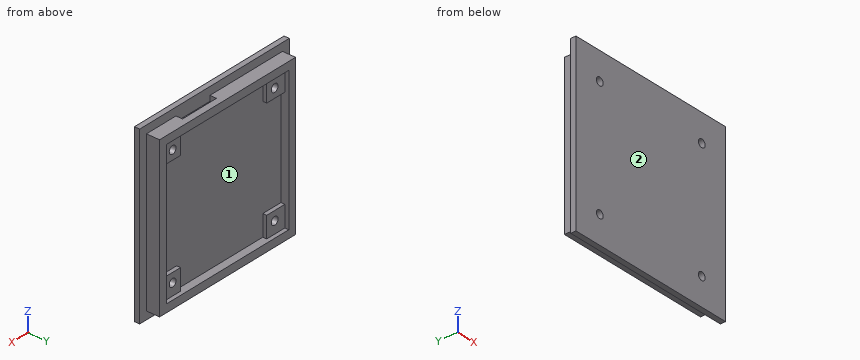
from build123d import *

# Parameters (mm, degrees)
SKETCH1_W           = 60
SKETCH1_H           = 60
BOSS_EXTRUDE1_DEPTH = 5
SKETCH2_W           = 54
SKETCH2_H           = 54
CUT_EXTRUDE1_DEPTH  = 3
SKETCH5_W           = 15
SKETCH5_H           = 2.5
CUT_EXTRUDE3_DEPTH  = 2
SKETCH6_W           = 12
SKETCH6_H           = 2
CUT_EXTRUDE4_DEPTH  = 2
SKETCH7_W           = 66
SKETCH7_H           = 66
BOSS_EXTRUDE3_DEPTH = 2
SKETCH4_W           = 8
SKETCH4_H           = 8
BOSS_EXTRUDE2_DEPTH = 1.5
SKETCH3_R           = 1.5
CUT_EXTRUDE2_DEPTH  = 5.5


with BuildPart() as part:
    # Sketch1 → Boss-Extrude1 (new body)
    with BuildSketch(Plane(origin=(0, 0, 0), x_dir=(1, 0, 0), z_dir=(0, 1, 0))):
        Rectangle(SKETCH1_W, SKETCH1_H)
    extrude(amount=BOSS_EXTRUDE1_DEPTH)

    # Sketch2 → Cut-Extrude1 (cut)
    with BuildSketch(Plane(origin=(0, 5, 0), x_dir=(1, 0, 0), z_dir=(0, 1, 0))):
        Rectangle(SKETCH2_W, SKETCH2_H)
    extrude(amount=-CUT_EXTRUDE1_DEPTH, mode=Mode.SUBTRACT)

    # Sketch5 → Cut-Extrude3 (cut)
    with BuildSketch(Plane(origin=(0, 0, 30), x_dir=(-1, 0, 0), z_dir=(0, 0, -1))):
        with Locations((-9.5, 1.25)):
            Rectangle(SKETCH5_W, SKETCH5_H)
    extrude(amount=CUT_EXTRUDE3_DEPTH, mode=Mode.SUBTRACT)

    # Sketch6 → Cut-Extrude4 (cut)
    with BuildSketch(Plane(origin=(0, 0, -30), x_dir=(-1, 0, 0), z_dir=(0, 0, -1))):
        with Locations((-17.5, 1)):
            Rectangle(SKETCH6_W, SKETCH6_H)
    extrude(amount=-CUT_EXTRUDE4_DEPTH, mode=Mode.SUBTRACT)

    # Sketch7 → Boss-Extrude3 (add)
    with BuildSketch(Plane.XZ):
        Rectangle(SKETCH7_W, SKETCH7_H)
    extrude(amount=BOSS_EXTRUDE3_DEPTH)

    # Sketch4 → Boss-Extrude2 (add)
    with BuildSketch(Plane(origin=(0, 2, 0), x_dir=(1, 0, 0), z_dir=(0, 1, 0))):
        with Locations((23, 23)):
            Rectangle(SKETCH4_W, SKETCH4_H)
        with Locations((-23, 23)):
            Rectangle(SKETCH4_W, SKETCH4_H)
        with Locations((23, -23)):
            Rectangle(SKETCH4_W, SKETCH4_H)
        with Locations((-23, -23)):
            Rectangle(SKETCH4_W, SKETCH4_H)
    extrude(amount=BOSS_EXTRUDE2_DEPTH)

    # Sketch3 → Cut-Extrude2 (cut)
    with BuildSketch(Plane(origin=(0, 3.5, 0), x_dir=(1, 0, 0), z_dir=(0, 1, 0))):
        with Locations(Location((-22.5, 22.5, 0), (0, 0, 270))):
            Circle(SKETCH3_R)
        with Locations(Location((22.5, 22.5, 0), (0, 0, 270))):
            Circle(SKETCH3_R)
        with Locations(Location((22.5, -22.5, 0), (0, 0, 270))):
            Circle(SKETCH3_R)
        with Locations(Location((-22.5, -22.5, 0), (0, 0, 270))):
            Circle(SKETCH3_R)
    extrude(amount=-CUT_EXTRUDE2_DEPTH, mode=Mode.SUBTRACT)


solid = part.part
Geometry check sheet. Reference: the model listing, model coordinates, mm. Face numbers are marked on the shaded views. Round coordinates to 2 decimals unless told otherwise and drop trailing zeros. Loops run counter-clockwise (first coordinate to the right, second up) from the corner with the lowest first, then second, coordinate; pieces in that order, holes last. Notation, with made-up numbers: (3.5, 89) - (11.5, 89) arc R33 cw to (11.5, 123) - close; hole circle Ø8 at (-24, 5.25). An arc over 180 degrees is marked (long way). One line per question, with ' | ' between items. Start each with the question number.
1. Draft check along Z on the marked faces 1 and 2. Enter one of: released by +Z, released by -Z, zero draft, split by the parting line, or undercut.
2. Cross-section at A-A on z = 22.5. Record the cut outline in (x, y).
3. Scan lines: line 1 (X direction, y = -0.2, z = -22.5); line 2 (X direction, y = 1.8, z = -22.5); line 3 (Z direction, x = -9.5, y = 4). Record each from-to range of solid material in increasing order. Write a range as [from, to].
4. Depth check by flat-ended pin: pin 1 (1 mm diameter, centred on y = 2, z = -2, fed in from -X); pin 2 (2.5 mm diameter, centred on x = 2.5, y = 4, fed in from +Z); pin 3 (1 mm diameter, centred on y = 2, z = -15, fed in from +X); pin 4 (9 mm diameter, centred on x = -23.5, z = -24, fed in from +Y). Enter the tip coordinate at first touch or a pass-through.
5. Cross-section at B-B on y = 0.75. Record the cut outline in (x, z), then the cut area to 3 significant figures.
6. Cross-section at C-C on x = -22.5. Record the cut outline in (y, z).
7. Cross-section at D-D on x = 3.5. Record the cut outline in (y, z).
Taken from the geometry:
1) face 1: undercut | face 2: zero draft
2) outline: (-33, -2) - (-24, -2) - (-24, 3.5) - (-27, 3.5) - (-27, 5) - (-30, 5) - (-30, 0) - (-33, 0) - close; (-21, -2) - (21, -2) - (21, 3.5) - (19, 3.5) - (19, 2) - (-19, 2) - (-19, 3.5) - (-21, 3.5) - close; (24, -2) - (33, -2) - (33, 0) - (30, 0) - (30, 5) - (27, 5) - (27, 3.5) - (24, 3.5) - close
3) line 1: [-33, -24], [-21, 21], [24, 33] | line 2: [-30, -24], [-21, 21], [24, 30] | line 3: [-30, -27], [27, 30]
4) pin 1: x = -30 | pin 2: z = 30 | pin 3: x = 30 | pin 4: y = 5
5) outline: (-30, -30) - (11.5, -30) - (11.5, -28) - (23.5, -28) - (23.5, -30) - (30, -30) - (30, 30) - (17, 30) - (17, 28) - (2, 28) - (2, 30) - (-30, 30) - close; hole circle Ø3 at (-22.5, -22.5); hole circle Ø3 at (-22.5, 22.5); hole circle Ø3 at (22.5, -22.5); hole circle Ø3 at (22.5, 22.5) | area: 3,520 mm²
6) outline: (-2, -33) - (0, -33) - (0, -30) - (5, -30) - (5, -27) - (3.5, -27) - (3.5, -24) - (-2, -24) - close; (-2, -21) - (3.5, -21) - (3.5, -19) - (2, -19) - (2, 19) - (3.5, 19) - (3.5, 21) - (-2, 21) - close; (-2, 24) - (3.5, 24) - (3.5, 27) - (5, 27) - (5, 30) - (0, 30) - (0, 33) - (-2, 33) - close
7) outline: (-2, -33) - (0, -33) - (0, -30) - (5, -30) - (5, -27) - (2, -27) - (2, 27) - (5, 27) - (5, 30) - (2.5, 30) - (2.5, 28) - (0, 28) - (0, 33) - (-2, 33) - close
